Autodesk Inventor part; units mm, degrees
ref_plane "YZ Plane" through (0, 0, 0) normal (1, 0, 0) x (0, 1, 0)
ref_plane "XZ Plane" through (0, 0, 0) normal (0, 1, 0) x (-1, 0, 0)
ref_plane "XY Plane" through (0, 0, 0) normal (0, 0, 1) x (1, 0, 0)
sketch "Sketch1" plane through (0, 0, 0) normal (0, 1, 0) x (-1, 0, 0)
  line L0 (0, 0) -> (-85, 0)
  line L1 (-85, 0) -> (-85, -56)
  line L2 (-85, -56) -> (0, -56)
  line L3 (0, -56) -> (0, 0)
  dimension "d0" = 85
  dimension "d1" = 56
extrude "Extrusion1" add sketch "Sketch1" along normal blind 1.8
fillet "Fillet1" radius 3 4 edges at (0, 0.9, 0) (85, 0.9, 0) (85, 0.9, -56) (0, 0.9, -56)
sketch "Sketch2" plane through (0, 1.8, 0) normal (0, 1, 0) x (1, 0, 0)
  line L0 (0, 53) -> (0, 3)
  line L1 (3, 0) -> (82, 0)
  line L2 (82, 56) -> (3, 56)
  point P0 (0, 0)
  point P1 (3.5, 52.5)
  point P2 (61.5, 52.5)
  point P3 (3.5, 3.5)
  point P4 (61.5, 3.5)
  dimension "d5" = 58
  dimension "d7" = 49
  dimension "d8" = 3.5
  dimension "d9" = 3.5
  dimension "d10" = 3.5
  dimension "d11" = 3.5
  dimension "d12" = 3.5
  dimension "d13" = 3.5
hole "Hole1" at (3.5, 1.8, -52.5) at (61.5, 1.8, -52.5) at (3.5, 1.8, -3.5) at (61.5, 1.8, -3.5) direction (0, -1, 0) diameter 3 end through all
sketch "Sketch3" plane through (0, 0, 0) normal (0, -1, 0) x (1, 0, 0)
  line L0 (0, -53) -> (0, -3)
  line L1 (14.2126, -21.7399) -> (0, -21.7399)
  line L2 (0, -21.7399) -> (0, -36.2099)
  line L3 (0, -36.2099) -> (14.2126, -36.2099)
  line L4 (14.2126, -36.2099) -> (14.2126, -21.7399)
  line L5 (41.7741, -5) -> (46.9065, -5)
  line L6 (46.9065, -5) -> (46.9065, -10.2381)
  line L7 (46.9065, -10.2381) -> (41.7741, -10.2381)
  line L8 (41.7741, -10.2381) -> (41.7741, -5)
  line L9 (58.8394, -15.3064) -> (64.9983, -15.3064)
  line L10 (64.9983, -15.3064) -> (64.9983, -21.337)
  line L11 (64.9983, -21.337) -> (58.8394, -21.337)
  line L12 (58.8394, -21.337) -> (58.8394, -15.3064)
  line L13 (56.1449, -39.6854) -> (63, -39.6854)
  line L14 (63, -39.6854) -> (63, -46.55)
  line L15 (63, -46.55) -> (56.1449, -46.55)
  line L16 (56.1449, -46.55) -> (56.1449, -39.6854)
  line L17 (30.8677, -14.7931) -> (45.8159, -29.4847)
  line L18 (45.8159, -29.4847) -> (31.0297, -44.5291)
  line L19 (31.0297, -44.5291) -> (16.0816, -29.8375)
  line L20 (16.0816, -29.8375) -> (30.8677, -14.7931)
  circle A0 centre (76.4179, -4.5925) radius 1.5529
  circle A1 centre (76.4179, -15.9302) radius 1.5186
  point P0 (0, 0)
extrude "Extrusion2" add sketch "Sketch3" along normal blind 1
sketch "Sketch4" plane through (0, 1.8, 0) normal (0, 1, 0) x (1, 0, 0)
  line L0 (6.6003, 22.2047) -> (20.4228, 22.2047)
  line L1 (20.4228, 22.2047) -> (20.4228, 10.4766)
  line L2 (20.4228, 10.4766) -> (6.6003, 10.4766)
  line L3 (6.6003, 10.4766) -> (6.6003, 22.2047)
  line L4 (44.413, 42.4767) -> (55.5812, 42.4767)
  line L5 (55.5812, 42.4767) -> (55.5812, 31.1828)
  line L6 (55.5812, 31.1828) -> (44.413, 31.1828)
  line L7 (44.413, 31.1828) -> (44.413, 42.4767)
  line L8 (44.413, 28.1626) -> (55.5812, 28.1626)
  line L9 (55.5812, 28.1626) -> (55.5812, 17.0574)
  line L10 (55.5812, 17.0574) -> (44.413, 17.0574)
  line L11 (44.413, 17.0574) -> (44.413, 28.1626)
  line L12 (57.5002, 34.8635) -> (66.4976, 34.8635)
  line L13 (66.4976, 34.8635) -> (66.4976, 25.9919)
  line L14 (66.4976, 25.9919) -> (57.5002, 25.9919)
  line L15 (57.5002, 25.9919) -> (57.5002, 34.8635)
  point P0 (0, 0)
extrude "Extrusion3" add sketch "Sketch4" along normal blind 1
sketch "Sketch5" plane through (0, 1.8, 0) normal (0, 1, 0) x (1, 0, 0)
  line L0 (3.0525, 45.1901) -> (5.1263, 45.1901)
  line L1 (5.1263, 45.1901) -> (5.1263, 24.9394)
  line L2 (5.1263, 24.9394) -> (3.0525, 24.9394)
  line L3 (3.0525, 24.9394) -> (3.0525, 45.1901)
  line L4 (7.8863, 45.1901) -> (9.9602, 45.1901)
  line L5 (9.9602, 45.1901) -> (9.9602, 24.9394)
  line L6 (9.9602, 24.9394) -> (7.8863, 24.9394)
  line L7 (7.8863, 24.9394) -> (7.8863, 45.1901)
  point P0 (0, 0)
  dimension "d25" = 0
extrude "Extrusion4" add sketch "Sketch5" along normal blind 3
sketch "Sketch6" plane through (0, 1.8, 0) normal (0, 1, 0) x (1, 0, 0)
  line L0 (41.9919, 16.3406) -> (47.3417, 16.3406)
  line L1 (47.3417, 16.3406) -> (47.3417, 0.8787)
  line L2 (47.3417, 0.8787) -> (41.9919, 0.8787)
  line L3 (41.9919, 0.8787) -> (41.9919, 16.3406)
  point P0 (0, 0)
extrude "Extrusion5" add sketch "Sketch6" along normal blind 5
properties part number "nanopi_m4_board"
The model under review builds one solid part; all positions refer to its coordinate system, in mm. A direction names the side the tool comes from. Round coordinates to 2 decimals unless told otherwise and drop trailing zeros. Loops run counter-clockwise (first coordinate to the right, second up) from the corner with the lowest first, then second, coordinate; pieces in that order, holes last.
1) The part is to be moulded in two halves that separate along X. For faces 1 (the face through (0, 1, -28)), 2 (the face through (4.4, 0.9, -53.7)), 3 (the face through (60, -1, -43)), say which applies: pulls with the +X half, pulls with the -X half, needs draft (parallel to the pull), parting line crosses it, or undercut.
Values follow:
face 1: pulls with the -X half
face 2: undercut
face 3: needs draft
2) Tool access review of faces 4 (the face through (38.2, -0.5, -22)), 5 (the face through (45, 4, -16.341)), 6 (the face through (4, 3, -45.19)): name each direction out of +Z, -Z, +X, -X, +Y, -Y from which nothing blocks a thin tool from reaching the whole face with its end or side.
Values follow:
face 4: -Y
face 5: +X, +Y
face 6: -Z, +X, -X, +Y
3) Consider section D-D on y = 5.75. State the section outline as (x, z) points.
Values follow:
outline: (41.99, -16.34) - (47.34, -16.34) - (47.34, -0.88) - (41.99, -0.88) - close
4) Wall thickness on line 1 along Z through (x, y) = (3.5, 1.25); line 2 along X through (y, z) = (0.5, -52.5); line 3 along X through (y, z) = (2.25, -32.5): over which ranges is each line inside the solid? List them lowest first.
Values follow:
line 1: z = -56 to -54, -51 to -5, -2 to 0
line 2: x = 0 to 2, 5 to 60, 63 to 85
line 3: x = 3.05 to 5.13, 7.89 to 9.96, 44.41 to 55.58, 57.5 to 66.5
5) Consider section C-C on x = 49.5. State the section outline as (y, z) points.
Values follow:
outline: (0, -56) - (1.8, -56) - (1.8, -42.48) - (2.8, -42.48) - (2.8, -31.18) - (1.8, -31.18) - (1.8, -28.16) - (2.8, -28.16) - (2.8, -17.06) - (1.8, -17.06) - (1.8, 0) - (0, 0) - close
6) Consider section B-B on z = -9. State the section outline as (x, y) points, then the cut area to 3 significant figures.
Values follow:
outline: (0, 0) - (41.77, 0) - (41.77, -1) - (46.91, -1) - (46.91, 0) - (85, 0) - (85, 1.8) - (47.34, 1.8) - (47.34, 6.8) - (41.99, 6.8) - (41.99, 1.8) - (0, 1.8) - close
area: 185 mm2
7) Clearance check with flat-ended pins moving along their axes: P1, Ø1, axis at x = 48, z = -9.5, coming from the +Y side; P2, Ø6, axis at x = 61.5, z = -30, coming from the +Y side; P3, Ø10, axis at x = 59, z = -31, coming from the -Y side; P4, Ø1.5, axis at y = 2.5, z = -39, coming from the +X side. State where each tip first meets the part, or that it passes through.
Values follow:
P1: stops at y = 1.8
P2: stops at y = 2.8
P3: stops at y = 0
P4: stops at x = 85
8) Consider section A-A on x = 61.5. State the section outline as (y, z) points.
Values follow:
outline: (-1, -46.55) - (0, -46.55) - (0, -51) - (1.8, -51) - (1.8, -34.86) - (2.8, -34.86) - (2.8, -25.99) - (1.8, -25.99) - (1.8, -5) - (0, -5) - (0, -15.31) - (-1, -15.31) - (-1, -21.34) - (0, -21.34) - (0, -39.69) - (-1, -39.69) - close; (0, -56) - (1.8, -56) - (1.8, -54) - (0, -54) - close; (0, -2) - (1.8, -2) - (1.8, 0) - (0, 0) - close
